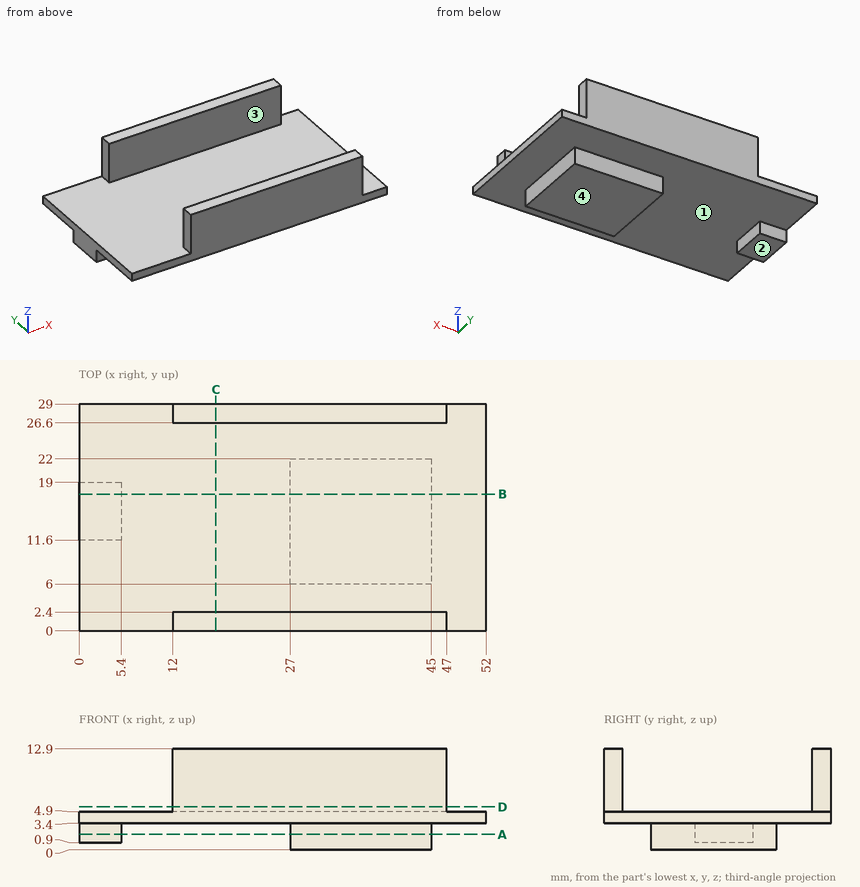
Verification items for this drawing (mm, ordinates from the low corner). A direction names the side the tool comes from. Give positions to 0.01 mm unless a question says otherwise; leave off trailing zeros. Loops run counter-clockwise (first coordinate to the right, second up) from the corner with the lowest first, then second, coordinate; pieces in that order, holes last.
(1) Set-up check for the marked faces 3 and 4: record each of +Z, -Z, +X, -X, +Y, -Y from which the full face is reachable in a straight line by a thin tool's end or side.
From the geometry:
face 3: +Z, +X, -X
face 4: -Z, +X, -X, +Y, -Y
(2) Depth check by flat-ended pin: pin 1 Ø1.7 at (x, z) = (39, 1.5) entering from -Y; pin 2 Ø3.5 at (x, z) = (40, 1) entering from +Y; pin 3 Ø2.5 at (y, z) = (13, 2) entering from +X; pin 4 Ø2.5 at (y, z) = (16, 1.5) entering from -X. Enter the tip coordinate at first touch or a pass-through.
From the geometry:
pin 1: stops at y = 6
pin 2: stops at y = 22
pin 3: stops at x = 45
pin 4: stops at x = 0
(3) Thickness scan on L1, parallel to Y at x = 27.5, z = 9.25; L2, parallel to Z at x = 3.5, y = 12.5; L3, parallel to X at y = 1.75, z = 8. Record the ranges inside material, lowest first.
From the geometry:
L1: y = 0 to 2.4, 26.6 to 29
L2: z = 0.9 to 4.9
L3: x = 12 to 47
(4) Section check B-B on y = 17.5. Record the cut outline in (x, z), then the cut area to 3 significant figures.
From the geometry:
outline: (0, 0.9) - (5.4, 0.9) - (5.4, 3.4) - (27, 3.4) - (27, 0) - (45, 0) - (45, 3.4) - (52, 3.4) - (52, 4.9) - (0, 4.9) - close
area: 153 mm2
(5) Release check for a two-part mould opening along X. For the marked faces 1 and 2 record: released by +X, released by -X, zero draft, split by the parting line, or undercut.
From the geometry:
face 1: undercut
face 2: zero draft
(6) Section check A-A on z = 2. Record the cut outline in (x, y), then the cut area to 3 significant figures.
From the geometry:
outline: (0, 11.6) - (5.4, 11.6) - (5.4, 19) - (0, 19) - close; (27, 6) - (45, 6) - (45, 22) - (27, 22) - close
area: 328 mm2
(7) Section check D-D on z = 5.5. Record the cut outline in (x, y).
From the geometry:
outline: (12, 0) - (47, 0) - (47, 2.4) - (12, 2.4) - close; (12, 26.6) - (47, 26.6) - (47, 29) - (12, 29) - close
(8) Section check C-C on x = 17.5. Record the cut outline in (y, z).
From the geometry:
outline: (0, 3.4) - (29, 3.4) - (29, 12.9) - (26.6, 12.9) - (26.6, 4.9) - (2.4, 4.9) - (2.4, 12.9) - (0, 12.9) - close
